The listing builds one solid part. Answer for the finished solid, in the listing's coordinates (mm). Coordinates: 2 decimals unless noted, no trailing zeros. Order: outer loops, then holes, each group sorted by start corner. A loop starts at its lowest first (then second) coordinate and runs counter-clockwise, first axis right, second up. Notation, with made-up numbers: (-23, 51) - (3, 51) arc R18 cw to (3, 69) - close; hole circle Ø5 at (82, 45.25). An arc over 180 degrees is marked (long way). Use one line per item in the form item = value. Start each with the question number.
Item 1: Section A-A, the plane x = 47 is taken. Write down the section's boundary in (y, z), and give its area (3 significant figures).
Item 2: Section B-B, the plane y = 60 is taken. Write down the section's boundary in (x, z).
Item 3: Section C-C, the plane z = 1.5 is taken. Count the separate pieces of the cut face and the enclosed holes in it, and give its area (3 significant figures).
Item 4: This flat-tipped pin is pushed along its axis until it touches: pin 1 Ø2.5 at (x, z) = (32, 3.5) entering from -Y. Where does it stop, or does it pass through?
Item 5: Consider line 1 along Y through (x, z) = (47, 3.25); line 2 along Y through (x, z) = (59.5, 1.6); line 3 along Y through (x, z) = (4, 3.6). Determine where each line is inside the solid, lowest interval first. Write a range as [from, to].
from build123d import *

# Parameters (mm, degrees)
SKETCH_1_R      = 2.5
SKETCH_1_W      = 8.9
SKETCH_1_H      = 19
EXTRUDE_1_DEPTH = 5


with BuildPart() as part:
    # 草图1 → 凸台-拉伸1 (new body)
    with BuildSketch(Plane.XY):
        with BuildLine():
            Line((3, 0), (25, 0))
            ThreePointArc((25, 0), (27.121320344, 0.878679656), (28, 3))
            Line((28, 3), (28, 5))
            Line((28, 5), (42, 5))
            Line((42, 5), (42, 3))
            ThreePointArc((42, 3), (42.878679656, 0.878679656), (45, 0))
            Line((45, 0), (67, 0))
            ThreePointArc((67, 0), (69.121320344, 0.878679656), (70, 3))
            Line((70, 3), (70, 25))
            ThreePointArc((70, 25), (69.121320344, 27.121320344), (67, 28))
            Line((67, 28), (65, 28))
            Line((65, 28), (65, 42))
            Line((65, 42), (67, 42))
            ThreePointArc((67, 42), (69.121320344, 42.878679656), (70, 45))
            Line((70, 45), (70, 67))
            ThreePointArc((70, 67), (69.121320344, 69.121320344), (67, 70))
            Line((67, 70), (45, 70))
            ThreePointArc((45, 70), (42.878679656, 69.121320344), (42, 67))
            Line((42, 67), (42, 65))
            Line((42, 65), (28, 65))
            Line((28, 65), (28, 67))
            ThreePointArc((28, 67), (27.121320344, 69.121320344), (25, 70))
            Line((25, 70), (3, 70))
            ThreePointArc((3, 70), (0.878679656, 69.121320344), (0, 67))
            Line((0, 67), (0, 45))
            ThreePointArc((0, 45), (0.878679656, 42.878679656), (3, 42))
            Line((3, 42), (5, 42))
            Line((5, 42), (5, 28))
            Line((5, 28), (3, 28))
            ThreePointArc((3, 28), (0.878679656, 27.121320344), (0, 25))
            Line((0, 25), (0, 3))
            ThreePointArc((0, 3), (0.878679656, 0.878679656), (3, 0))
        make_face()
        with Locations((23, 47)):
            Circle(SKETCH_1_R, mode=Mode.SUBTRACT)
        with Locations((47, 47)):
            Circle(SKETCH_1_R, mode=Mode.SUBTRACT)
        with Locations((23, 23)):
            Circle(SKETCH_1_R, mode=Mode.SUBTRACT)
        with Locations((47, 23)):
            Circle(SKETCH_1_R, mode=Mode.SUBTRACT)
        with Locations((63.55, 56.5)):
            Rectangle(SKETCH_1_W, SKETCH_1_H, mode=Mode.SUBTRACT)
        with Locations((63.55, 13.5)):
            Rectangle(SKETCH_1_W, SKETCH_1_H, mode=Mode.SUBTRACT)
        with Locations((6.45, 56.5)):
            Rectangle(SKETCH_1_W, SKETCH_1_H, mode=Mode.SUBTRACT)
        with Locations((6.45, 13.5)):
            Rectangle(SKETCH_1_W, SKETCH_1_H, mode=Mode.SUBTRACT)
    extrude(amount=EXTRUDE_1_DEPTH)


solid = part.part
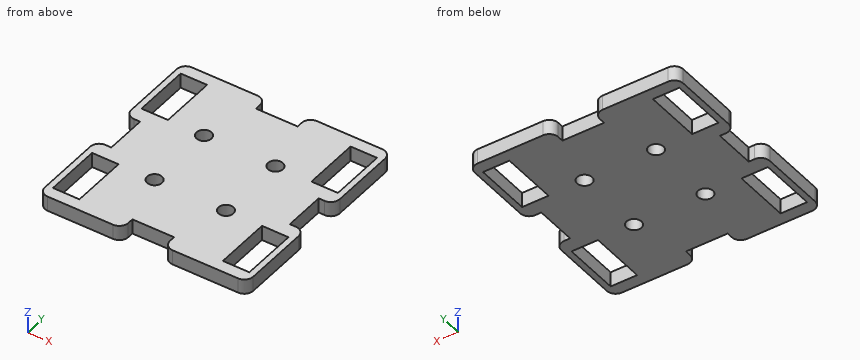
Response:
q1.outline = (0, 0) - (20.5, 0) - (20.5, 5) - (0, 5) - close; (25.5, 0) - (44.5, 0) - (44.5, 5) - (25.5, 5) - close; (49.5, 0) - (70, 0) - (70, 5) - (49.5, 5) - close
q1.area = 300 mm2
q2.outline = (0, 0) - (2, 0) - (2, 5) - (0, 5) - close; (10.9, 0) - (59.1, 0) - (59.1, 5) - (10.9, 5) - close; (68, 0) - (70, 0) - (70, 5) - (68, 5) - close
q3.separate_pieces = 1
q3.enclosed_holes = 8
q3.area = 3,840 mm2
q4.pin_1 = 5
q5.line_1 = [0, 20.5], [25.5, 44.5], [49.5, 70]
q5.line_2 = [0, 4], [23, 47], [66, 70]
q5.line_3 = [0, 4], [23, 28], [42, 47], [66, 70]
